Model file for the job. Use its own axes, mm. A direction names the side the tool comes from. Coordinates: 2 decimals unless noted, no trailing zeros. Order: outer loops, then holes, each group sorted by start corner. A loop starts at its lowest first (then second) coordinate and runs counter-clockwise, first axis right, second up.
from build123d import *

# Parameters (mm, degrees)
ESQUISSE1_R             = 5
BOSS_EXTRU_1_DEPTH      = 5
ESQUISSE2_R             = 2.5
BOSS_EXTRU_2_DEPTH      = 5
ESQUISSE3_R             = 1.5
ENL_V_MAT_EXTRU_2_DEPTH = 5
ESQUISSE4_R             = 2.05
ENL_V_MAT_EXTRU_3_DEPTH = 5


with BuildPart() as part:
    # Esquisse1 → Boss.-Extru.1 (new body)
    with BuildSketch(Plane(origin=(0, 0, 0), x_dir=(1, 0, 0), z_dir=(0, 1, 0))):
        with Locations(Location((0, 0, 0), (0, 0, 270))):
            Circle(ESQUISSE1_R)
    extrude(amount=BOSS_EXTRU_1_DEPTH)

    # Esquisse2 → Boss.-Extru.2 (add)
    with BuildSketch(Plane(origin=(0, 5, 0), x_dir=(1, 0, 0), z_dir=(0, 1, 0))):
        with Locations(Location((0, 0, 0), (0, 0, 270))):
            Circle(ESQUISSE2_R)
    extrude(amount=BOSS_EXTRU_2_DEPTH)

    # Esquisse3 → Enlèv. mat.-Extru.2 (cut)
    with BuildSketch(Plane(origin=(0, 10, 0), x_dir=(1, 0, 0), z_dir=(0, 1, 0))):
        with Locations(Location((0, 0, 0), (0, 0, 270))):
            Circle(ESQUISSE3_R)
    extrude(amount=-ENL_V_MAT_EXTRU_2_DEPTH, mode=Mode.SUBTRACT)

    # Esquisse4 → Enlèv. mat.-Extru.3 (cut)
    with BuildSketch(Plane.XZ):
        with Locations(Location((0, 0, 0), (0, 0, 270))):
            Circle(ESQUISSE4_R)
    extrude(amount=-ENL_V_MAT_EXTRU_3_DEPTH, mode=Mode.SUBTRACT)


solid = part.part
Q1. Drop flat-ended pins along their axis: P1, Ø4, axis at y = 1.5, z = 1, coming from the +X side; P2, Ø2, axis at y = 7.5, z = -3, coming from the +X side; P3, Ø1.5, axis at x = 0, z = 4, coming from the +Y side. Give the stop position or say it passes through.
Established:
P1: stops at x = 5
P2: stops at x = 1.5
P3: stops at y = 5
Q2. Cut at D-D, the plane x = 1.75. List the corners of the cut face in (y, z), plus the area to 3 significant figures.
Established:
outline: (0, -4.68) - (5, -4.68) - (5, -1.79) - (10, -1.79) - (10, 1.79) - (5, 1.79) - (5, 4.68) - (0, 4.68) - (0, 1.07) - (5, 1.07) - (5, -1.07) - (0, -1.07) - close
area: 54.0 mm2
Q3. Cut at A-A, the plane x = 0. List the corners of the cut face in (y, z).
Established:
outline: (0, -5) - (5, -5) - (5, -2.5) - (10, -2.5) - (10, -1.5) - (5, -1.5) - (5, -2.05) - (0, -2.05) - close; (0, 2.05) - (5, 2.05) - (5, 1.5) - (10, 1.5) - (10, 2.5) - (5, 2.5) - (5, 5) - (0, 5) - close
Q4. Cut at C-C, the plane y = 3.5. List the corners of the cut face in (x, z).
Established:
outline: circle Ø10 at (0, 0); hole circle Ø4.1 at (0, 0)
Q5. Cut at B-B, the plane z = 0. List the corners of the cut face in (x, y), plus the area to 3 significant figures.
Established:
outline: (-5, 0) - (-2.05, 0) - (-2.05, 5) - (-1.5, 5) - (-1.5, 10) - (-2.5, 10) - (-2.5, 5) - (-5, 5) - close; (1.5, 5) - (2.05, 5) - (2.05, 0) - (5, 0) - (5, 5) - (2.5, 5) - (2.5, 10) - (1.5, 10) - close
area: 39.5 mm2
Q6. Probe line 1 (X direction, y = 3.45, z = 0); line 2 (X direction, y = 8.5, z = 0); line 3 (Y direction, x = 2.75, z = 0.5). List the from-to ranges inside material, lowest first.
Established:
line 1: x = -5 to -2.05, 2.05 to 5
line 2: x = -2.5 to -1.5, 1.5 to 2.5
line 3: y = 0 to 5
Q7. Mould opens along Z. For faces 4 (the face through (0.45, 7.54, 1.43)), 5 (the face through (-4.88, 2.46, -1.08)), 6 (the face through (-2, 10, 0)) say: pulls with the +Z half, pulls with the -Z half, needs draft (parallel to the pull), parting line crosses it, or undercut.
Established:
face 4: undercut
face 5: parting line crosses it
face 6: needs draft
Q8. Which spindle directions (+Z, -Z, +X, -X, +Y, -Y) get a long thin tool onto all of the face, cutting with end or side? Do faces 1 (the face through (-2, 5, 2)), 2 (the face through (0.1, 0, 2.2)), 3 (the face through (2.033, 2.465, 0.267)). Say none if no direction does.
Established:
face 1: +Y
face 2: +Z, -Z, +X, -X, -Y
face 3: -Y
